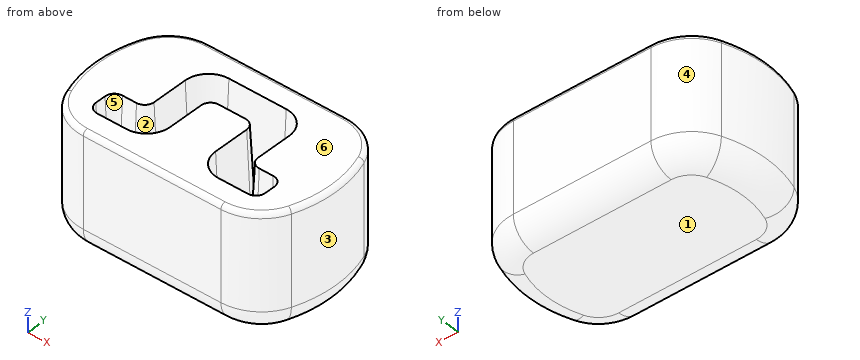
```python
from build123d import *

# Parameters (mm, degrees)
F1_DEPTH = 25
F2_DEPTH = 20
F2_TAPER = 3
F3_R     = 1
F4_R     = 5


with BuildPart() as f1:
    # F0 (on Top) → F1 (new body)
    with BuildSketch(Plane.XY):
        with BuildLine():
            ThreePointArc((-14.723294392, 15.45), (-20.4366897043, 13.6571379912), (-24.1014191371, 8.9214228012))
            ThreePointArc((-24.1014191371, 8.9214228012), (-25.6996145734, 0), (-24.1014191371, -8.9214228012))
            ThreePointArc((-24.1014191371, -8.9214228012), (-20.4366897043, -13.6571379912), (-14.723294392, -15.45))
            Line((-14.723294392, -15.45), (14.723294392, -15.45))
            ThreePointArc((14.723294392, -15.45), (20.4366897043, -13.6571379912), (24.1014191371, -8.9214228012))
            ThreePointArc((24.1014191371, -8.9214228012), (25.6996145734, 0), (24.1014191371, 8.9214228012))
            ThreePointArc((24.1014191371, 8.9214228012), (20.4366897043, 13.6571379912), (14.723294392, 15.45))
            Line((14.723294392, 15.45), (-14.723294392, 15.45))
        make_face()
        with BuildLine():
            Line((-6.125, 10.45), (6.125, 10.45))
            ThreePointArc((6.125, 10.45), (9.6605339059, 8.9855339059), (11.125, 5.45))
            Line((11.125, 5.45), (11.125, -2.2))
            ThreePointArc((11.125, -2.2), (11.7107864376, -3.6142135624), (13.125, -4.2))
            Line((13.125, -4.2), (16.125, -4.2))
            ThreePointArc((16.125, -4.2), (17.5392135624, -4.7857864376), (18.125, -6.2))
            Line((18.125, -6.2), (18.125, -8.45))
            ThreePointArc((18.125, -8.45), (17.5392135624, -9.8642135624), (16.125, -10.45))
            Line((16.125, -10.45), (9.875, -10.45))
            ThreePointArc((9.875, -10.45), (6.3394660941, -8.9855339059), (4.875, -5.45))
            Line((4.875, -5.45), (4.875, 2.2))
            ThreePointArc((4.875, 2.2), (4.2892135624, 3.6142135624), (2.875, 4.2))
            Line((2.875, 4.2), (-2.875, 4.2))
            ThreePointArc((-2.875, 4.2), (-4.2892135624, 3.6142135624), (-4.875, 2.2))
            Line((-4.875, 2.2), (-4.875, -5.45))
            ThreePointArc((-4.875, -5.45), (-6.3394660941, -8.9855339059), (-9.875, -10.45))
            Line((-9.875, -10.45), (-16.125, -10.45))
            ThreePointArc((-16.125, -10.45), (-17.5392135624, -9.8642135624), (-18.125, -8.45))
            Line((-18.125, -8.45), (-18.125, -6.2))
            ThreePointArc((-18.125, -6.2), (-17.5392135624, -4.7857864376), (-16.125, -4.2))
            Line((-16.125, -4.2), (-13.125, -4.2))
            ThreePointArc((-13.125, -4.2), (-11.7107864376, -3.6142135624), (-11.125, -2.2))
            Line((-11.125, -2.2), (-11.125, 5.45))
            ThreePointArc((-11.125, 5.45), (-9.6605339059, 8.9855339059), (-6.125, 10.45))
        make_face(mode=Mode.SUBTRACT)
        with BuildLine():
            ThreePointArc((11.125, 5.45), (9.6605339059, 8.9855339059), (6.125, 10.45))
            Line((6.125, 10.45), (-6.125, 10.45))
            ThreePointArc((-6.125, 10.45), (-9.6605339059, 8.9855339059), (-11.125, 5.45))
            Line((-11.125, 5.45), (-11.125, -2.2))
            ThreePointArc((-11.125, -2.2), (-11.7107864376, -3.6142135624), (-13.125, -4.2))
            Line((-13.125, -4.2), (-16.125, -4.2))
            ThreePointArc((-16.125, -4.2), (-17.5392135624, -4.7857864376), (-18.125, -6.2))
            Line((-18.125, -6.2), (-18.125, -8.45))
            ThreePointArc((-18.125, -8.45), (-17.5392135624, -9.8642135624), (-16.125, -10.45))
            Line((-16.125, -10.45), (-9.875, -10.45))
            ThreePointArc((-9.875, -10.45), (-6.3394660941, -8.9855339059), (-4.875, -5.45))
            Line((-4.875, -5.45), (-4.875, 2.2))
            ThreePointArc((-4.875, 2.2), (-4.2892135624, 3.6142135624), (-2.875, 4.2))
            Line((-2.875, 4.2), (2.875, 4.2))
            ThreePointArc((2.875, 4.2), (4.2892135624, 3.6142135624), (4.875, 2.2))
            Line((4.875, 2.2), (4.875, -5.45))
            ThreePointArc((4.875, -5.45), (6.3394660941, -8.9855339059), (9.875, -10.45))
            Line((9.875, -10.45), (16.125, -10.45))
            ThreePointArc((16.125, -10.45), (17.5392135624, -9.8642135624), (18.125, -8.45))
            Line((18.125, -8.45), (18.125, -6.2))
            ThreePointArc((18.125, -6.2), (17.5392135624, -4.7857864376), (16.125, -4.2))
            Line((16.125, -4.2), (13.125, -4.2))
            ThreePointArc((13.125, -4.2), (11.7107864376, -3.6142135624), (11.125, -2.2))
            Line((11.125, -2.2), (11.125, 5.45))
        make_face()
    extrude(amount=-F1_DEPTH)

    # F0 (on Top) → F2 (cut)
    with BuildSketch(Plane.XY):
        with BuildLine():
            ThreePointArc((11.125, 5.45), (9.6605339059, 8.9855339059), (6.125, 10.45))
            Line((6.125, 10.45), (-6.125, 10.45))
            ThreePointArc((-6.125, 10.45), (-9.6605339059, 8.9855339059), (-11.125, 5.45))
            Line((-11.125, 5.45), (-11.125, -2.2))
            ThreePointArc((-11.125, -2.2), (-11.7107864376, -3.6142135624), (-13.125, -4.2))
            Line((-13.125, -4.2), (-16.125, -4.2))
            ThreePointArc((-16.125, -4.2), (-17.5392135624, -4.7857864376), (-18.125, -6.2))
            Line((-18.125, -6.2), (-18.125, -8.45))
            ThreePointArc((-18.125, -8.45), (-17.5392135624, -9.8642135624), (-16.125, -10.45))
            Line((-16.125, -10.45), (-9.875, -10.45))
            ThreePointArc((-9.875, -10.45), (-6.3394660941, -8.9855339059), (-4.875, -5.45))
            Line((-4.875, -5.45), (-4.875, 2.2))
            ThreePointArc((-4.875, 2.2), (-4.2892135624, 3.6142135624), (-2.875, 4.2))
            Line((-2.875, 4.2), (2.875, 4.2))
            ThreePointArc((2.875, 4.2), (4.2892135624, 3.6142135624), (4.875, 2.2))
            Line((4.875, 2.2), (4.875, -5.45))
            ThreePointArc((4.875, -5.45), (6.3394660941, -8.9855339059), (9.875, -10.45))
            Line((9.875, -10.45), (16.125, -10.45))
            ThreePointArc((16.125, -10.45), (17.5392135624, -9.8642135624), (18.125, -8.45))
            Line((18.125, -8.45), (18.125, -6.2))
            ThreePointArc((18.125, -6.2), (17.5392135624, -4.7857864376), (16.125, -4.2))
            Line((16.125, -4.2), (13.125, -4.2))
            ThreePointArc((13.125, -4.2), (11.7107864376, -3.6142135624), (11.125, -2.2))
            Line((11.125, -2.2), (11.125, 5.45))
        make_face()
    extrude(amount=-F2_DEPTH, taper=F2_TAPER, mode=Mode.SUBTRACT)

    # F3
    f3_edges = [f1.edges().sort_by_distance(p)[0] for p in [
        (0, -15.45, 0),
    ]]
    fillet(f3_edges, radius=F3_R)

    # F4
    f4_edges = [f1.edges().sort_by_distance(p)[0] for p in [
        (0, -15.45, -25),
    ]]
    fillet(f4_edges, radius=F4_R)


solid = f1.part
```
Design review of the part built by this model. Coordinates are the model's own, in mm. Face numbers are marked on the shaded views. A direction names the side the tool comes from. Give positions to 0.01 mm unless a question says otherwise; leave off trailing zeros. One line per item, written item: value.
Q1. Draft analysis for pull direction X (two halves, no side actions). For the marked faces 3, 4, 5 and 6, state which applies: pulls with the +X half, pulls with the -X half, needs draft (parallel to the pull), parting line crosses it, or undercut.
Numbers:
face 3: pulls with the +X half
face 4: pulls with the -X half
face 5: undercut
face 6: needs draft
Q2. For L1, parallel to X at y = -5.5, z = -6; L2, parallel to X at y = -0.5, z = -17.75; L3, parallel to Y at x = -12.5, z = -7, list the stretches that pass through material, from the lowest coordinate up.
Numbers:
L1: x = -25.1 to -17.66, -5.19 to 5.19, 17.66 to 25.1
L2: x = -25.69 to -10.19, -5.81 to 5.81, 10.19 to 25.69
L3: y = -15.45 to -10.08, -4.48 to 15.45
Q3. For pin 1 Ø2 at (x, y) = (8, 12) entering from -Z; pin 2 Ø1.5 at (x, y) = (-4.5, 0) entering from +Z; pin 3 Ø5 at (x, z) = (-19.5, -5.5) entering from +Y; pin 4 Ø5 at (y, z) = (4.5, -8) entering from +X, all flat-tipped, find the tip position at first contact; note any pin that passes through.
Numbers:
pin 1: stops at z = -24.97
pin 2: stops at z = 0
pin 3: stops at y = 15.19
pin 4: stops at x = 25.62
Q4. Machinability: for the marked faces 1 and 2, which of the approach directions +Z, -Z, +X, -X, +Y, -Y give a long, thin tool a straight path to every point of the face, cutting with its end or side? Answer none if there is none.
Numbers:
face 1: -Z, +X, -X, +Y, -Y
face 2: +Z
